Source: three-view drawing plus pictorial views. Frame: mm from the lowest corner of the part. Give positions to 0.01 mm unless a question says otherwise; leave off trailing zeros. Order: outer loops, then holes, each group sorted by start corner. A loop starts at its lowest first (then second) coordinate and runs counter-clockwise, first axis right, second up. Notation, with made-up numbers: (-27, 52) - (5, 52) arc R4 cw to (5, 58) - close; hole circle Ø3 at (61.5, 13.5). An arc over 180 degrees is marked (long way). Use CSV: the item, a comma, the result in double quotes.
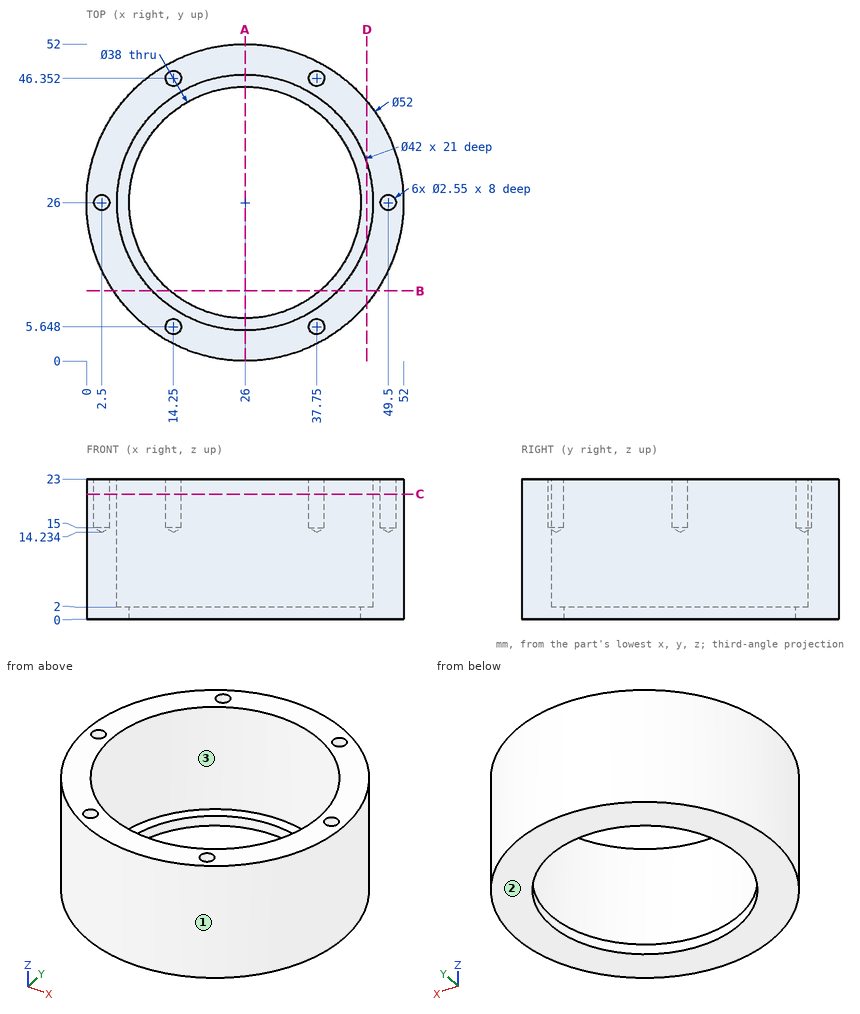
Item 1: Section A-A on x = 26. Return the cut outline in (y, z), then the cut area to 3 significant figures.
Filled in:
outline,"(0, 0) - (7, 0) - (7, 2) - (5, 2) - (5, 23) - (0, 23) - close; (45, 0) - (52, 0) - (52, 23) - (47, 23) - (47, 2) - (45, 2) - close"
area,"238 mm2"
Item 2: Section B-B on y = 11.5. Return the cut outline in (x, z), then the cut area to 3 significant figures.
Filled in:
outline,"(4.42, 0) - (13.72, 0) - (13.72, 2) - (10.81, 2) - (10.81, 23) - (4.42, 23) - close; (38.28, 0) - (47.58, 0) - (47.58, 23) - (41.19, 23) - (41.19, 2) - (38.28, 2) - close"
area,"306 mm2"
Item 3: Section D-D on x = 46. Return the cut outline in (y, z), then the cut area to 3 significant figures.
Filled in:
outline,"(9.39, 0) - (42.61, 0) - (42.61, 23) - (32.4, 23) - (32.4, 2) - (19.6, 2) - (19.6, 23) - (9.39, 23) - close"
area,"495 mm2"
Item 4: First-contact query: pin 1 (2 mm diameter, centred on x = 9, z = 8, fed in from +Y) (1 decimal); pin 2 (6 mm diameter, centred on x = 14.5, z = 5, fed in from -Y); pin 3 (4 mm diameter, centred on x = 32.5, z = 12.5, fed in from +Y). Flat tips, straight axial feed; report the tip coordinate or a pass-through.
Filled in:
pin 1,"stops at y = 46.5"
pin 2,"stops at y = 1.43"
pin 3,"stops at y = 51.61"
Item 5: Section C-C on z = 20.5. Count the separate pieces of the cut face and the enclosed holes in it.
Filled in:
separate pieces,"1"
enclosed holes,"7"
Item 6: Material intervals for line 1 (X direction, y = 26, z = 16) (1 decimal); line 2 (X direction, y = 26, z = 0.85); line 3 (X direction, y = 34, z = 18.75), sorted ascending. Write a range as from..to.
Filled in:
line 1,"x = 0..1.2, 3.8..5, 47..48.2, 50.8..52"
line 2,"x = 0..7, 45..52"
line 3,"x = 1.26..6.58, 45.42..50.74"
Item 7: Mould query, pull axis Y, two halves, no side actions, for the marked faces 1, 2 and 3. Classes: released by +Y, released by -Y, zero draft, split by the parting line, or undercut.
Filled in:
face 1,"split by the parting line"
face 2,"zero draft"
face 3,"undercut"
